Model file for the job. Use its own axes, mm. Face numbers are marked on the shaded views. A direction names the side the tool comes from. Coordinates: 2 decimals unless noted, no trailing zeros. Loops run counter-clockwise (first coordinate to the right, second up) from the corner with the lowest first, then second, coordinate; pieces in that order, holes last. Notation, with made-up numbers: M 75.5,52.5 L 118.5,52.5 A22 ccw 118.5,79.5 Z; hole C 84,-25 d6. An arc over 180 degrees is marked long. Write item = value, one per line. Start each with the question number.
Autodesk Inventor part; units mm, degrees
ref_plane "YZ Plane" through (0, 0, 0) normal (1, 0, 0) x (0, 1, 0)
ref_plane "XZ Plane" through (0, 0, 0) normal (0, 1, 0) x (-1, 0, 0)
ref_plane "XY Plane" through (0, 0, 0) normal (0, 0, 1) x (1, 0, 0)
sketch "Sketch1" plane through (0, 0, 0) normal (0, 0, 1) x (1, 0, 0)
  line L0 (-19, -19) -> (19, -19)
  line L1 (19, -19) -> (19, 19)
  line L2 (19, 19) -> (-19, 19)
  line L3 (-19, 19) -> (-19, -19)
  line L4 (-19, -19) -> (19, 19) construction
  line L5 (19, -19) -> (-19, 19) construction
  point P0 (0, 0)
  dimension "d0" = 38
extrude "Extrusion1" add sketch "Sketch1" along normal blind 100
sketch "Sketch2" plane through (0, 0, 0) normal (0, 0, -1) x (-1, 0, 0)
  circle A0 centre (0, 0) radius 16.15
  dimension "d3" = 32.3
extrude "Extrusion2" cut sketch "Sketch2" against normal blind 32
sketch "Sketch3" plane through (0, 0, 100) normal (0, 0, 1) x (1, 0, 0)
  circle A0 centre (0, 0) radius 17
  dimension "d6" = 34
extrude "Extrusion3" cut sketch "Sketch3" against normal blind 60
sketch "Sketch4" plane through (0, 0, 40) normal (0, 0, 1) x (1, 0, 0)
  circle A0 centre (0, 0) radius 10
  dimension "d9" = 20
extrude "Extrusion4" cut sketch "Sketch4" against normal through all
sketch "Sketch5" plane through (0, 0, 40) normal (0, 0, 1) x (1, 0, 0)
  point P0 (0, 0)
  point P1 (0, 13)
  dimension "d12" = 13
hole "Hole1" at (0, 13, 40) direction (0, 0, -1) diameter 3.4 end through all countersink diameter 7.5 countersink angle 90
pattern_circular "Circular Pattern1" count 4 over 360 about axis through (0, 0, -10) along (0, 0, 1) of "Hole1"
sketch "Sketch6" plane through (0, 0, 100) normal (0, 0, 1) x (1, 0, 0)
  line L0 (26.1087, -24.9255) -> (-24.3734, -24.9255)
  line L1 (-24.3734, -24.9255) -> (-24.3734, 25.8721)
  line L2 (-24.3734, 25.8721) -> (26.1087, 25.8721)
  line L3 (26.1087, 25.8721) -> (26.1087, -24.9255)
  point P0 (0, 0)
extrude "Extrusion5" cut sketch "Sketch6" against normal up to surface (60 mm away)
sketch "Sketch7" plane through (0, 0, 0) normal (0, 0, -1) x (-1, 0, 0)
  line L0 (21.4324, -23.2888) -> (-21.2074, -23.2888)
  line L1 (-21.2074, -23.2888) -> (-21.2074, 21.7137)
  line L2 (-21.2074, 21.7137) -> (21.4324, 21.7137)
  line L3 (21.4324, 21.7137) -> (21.4324, -23.2888)
  point P0 (0, 0)
extrude "Extrusion6" cut sketch "Sketch7" against normal blind 22.75
properties part number "402-gearbox-housing"
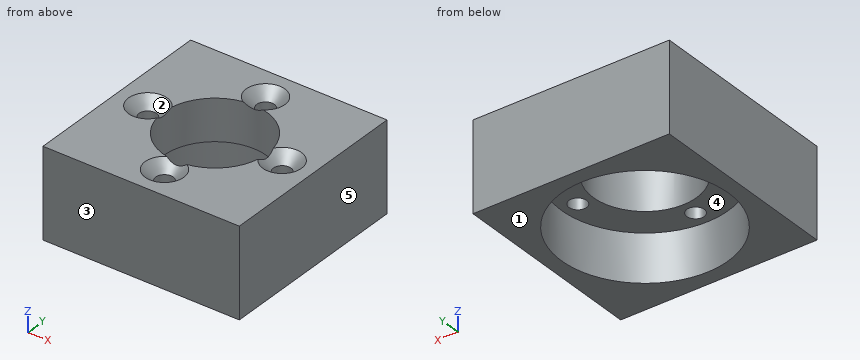
Item 1: 3-axis set-ups, long thin cutter, end or side, ignore diameter. For the marked faces 4 and 5: which of +Z, -Z, +X, -X, +Y, -Y reach the whole face in a straight line?
Item 2: Cut at C-C (z = 24.75). Give the cut face in (x, y).
Item 3: Pull direction Y, two halves, no side cores. Call the marked faces 1, 2 and 3: +Y half, -Y half, draft (parallel to the pull), parting line (faces both ways), or undercut.
Item 4: Cut at A-A (y = 0). Give the cut face in (x, z).
Item 5: Pin check, flat tips, straight feed: pin 1 Ø9.5 at (x, y) = (-4, 3.5) entering from -Z; pin 2 Ø4.5 at (x, y) = (0, 13) entering from +Z. Stop position of each tip, or through.
Item 6: Probe L1, parallel to X at y = 2, z = 32.5; L2, parallel to Y at x = 0, z = 27.25; L3, parallel to Y at x = -13, z = 36.1. List the from-to ranges inside material, lowest first.
Item 7: Cut at B-B (x = 13). Give the cut face in (y, z), plus the area to 3 significant figures.
Reported:
q1.face_4 = -Z
q1.face_5 = +Z, -Z, +X, +Y, -Y
q2.outline = M -19,-19 L 19,-19 L 19,19 L -19,19 Z; hole C 0,0 d32.3
q3.face_1 = draft
q3.face_2 = undercut
q3.face_3 = -Y half
q4.outline = M -19,22.75 L -16.15,22.75 L -16.15,32 L -14.7,32 L -14.7,37.95 L -16.75,40 L -19,40 Z; M -11.3,32 L -10,32 L -10,39.25 L -11.3,37.95 Z; M 10,32 L 11.3,32 L 11.3,37.95 L 10,39.25 Z; M 14.7,32 L 16.15,32 L 16.15,22.75 L 19,22.75 L 19,40 L 16.75,40 L 14.7,37.95 Z
q5.pin_1 = 32
q5.pin_2 = 38.5
q6.L1 = -19 to -9.8, 9.8 to 19
q6.L2 = -19 to -16.15, 16.15 to 19
q6.L3 = -19 to -1.7, 1.7 to 19
q7.outline = M -19,22.75 L -9.58,22.75 L -9.58,32 L -1.7,32 L -1.7,37.95 L -3.75,40 L -19,40 Z; M 1.7,32 L 9.58,32 L 9.58,22.75 L 19,22.75 L 19,40 L 3.75,40 L 1.7,37.95 Z
q7.area = 447 mm^2
